Read the model definition and answer for the solid it produces. Units are mm, in the model's axes. A direction names the side the tool comes from. Coordinates: 2 decimals unless noted, no trailing zeros. Loops run counter-clockwise (first coordinate to the right, second up) from the corner with the lowest first, then second, coordinate; pieces in that order, holes last.
from build123d import *

# Parameters (mm, degrees)
CYLINDER004_R          = 1.5
CYLINDER004_DEPTH      = 10
CYLINDER004_ROLL_ANGLE = 90
CYLINDER003_R          = 1.5
CYLINDER003_DEPTH      = 10
CYLINDER003_ROLL_ANGLE = 90
BOX016_W               = 22.5
BOX016_H               = 13
BOX016_DEPTH           = 13
BOX015_W               = 38
BOX015_H               = 10
BOX015_DEPTH           = 13
BOX013_W               = 98.5
BOX013_H               = 62
BOX013_DEPTH           = 10
BOX012_W               = 114.5
BOX012_H               = 66
BOX012_DEPTH           = 4
BOX014_W               = 118.5
BOX014_H               = 70
BOX014_DEPTH           = 5
BOX010_W               = 2
BOX010_H               = 10
BOX010_DEPTH           = 8
BOX010_PLACEMENT_ANGLE = 59
BOX011_W               = 2
BOX011_H               = 10
BOX011_DEPTH           = 8
BOX011_PLACEMENT_ANGLE = 59
BOX009_W               = 2
BOX009_H               = 10
BOX009_DEPTH           = 8
BOX009_PLACEMENT_ANGLE = 59
BOX008_W               = 2
BOX008_H               = 10
BOX008_DEPTH           = 8
BOX008_PLACEMENT_ANGLE = 59
BOX007_W               = 10
BOX007_H               = 45
BOX007_DEPTH           = 50
BOX006_W               = 14
BOX006_H               = 12
BOX006_DEPTH           = 12
BOX006_PLACEMENT_ANGLE = 59
BOX004_W               = 14
BOX004_H               = 12
BOX004_DEPTH           = 12
BOX004_PLACEMENT_ANGLE = 59
BOX002_W               = 71
BOX002_H               = 10
BOX002_DEPTH           = 25
BOX001_W               = 80
BOX001_H               = 30
BOX001_DEPTH           = 50
BOX_W                  = 84
BOX_H                  = 30
BOX_DEPTH              = 70
CYLINDER001_R          = 70
CYLINDER001_DEPTH      = 87
CYLINDER_R             = 72.5
CYLINDER_DEPTH         = 80
CYLINDER002_R          = 68
CYLINDER002_DEPTH      = 85


with BuildPart() as screwcutout002:
    # Cylinder004 → Cylinder004 (new body)
    with BuildSketch(Plane.XY):
        Circle(CYLINDER004_R)
    extrude(amount=CYLINDER004_DEPTH)


with BuildPart() as screwcutout002_1:
    # Cylinder004 roll: moved
    add(screwcutout002.part.rotate(Axis((0, 0, 0), (1, 0, 0)), CYLINDER004_ROLL_ANGLE))


with BuildPart() as screwcutout002_2:
    # Cylinder004 placement: moved
    add(screwcutout002_1.part.moved(Location((-15, 73, 14.5))))


with BuildPart() as screwcutout1:
    # Cylinder003 → Cylinder003 (new body)
    with BuildSketch(Plane.XY):
        Circle(CYLINDER003_R)
    extrude(amount=CYLINDER003_DEPTH)


with BuildPart() as screwcutout1_1:
    # Cylinder003 roll: moved
    add(screwcutout1.part.rotate(Axis((0, 0, 0), (1, 0, 0)), CYLINDER003_ROLL_ANGLE))


with BuildPart() as screwcutout1_2:
    # Cylinder003 placement: moved
    add(screwcutout1_1.part.moved(Location((15, 73, 14.5))))


with BuildPart() as powercutout:
    # Box016 → Box016 (new body)
    with BuildSketch(Plane(origin=(-11.25, 63, 8), x_dir=(1, 0, 0), z_dir=(0, 0, 1))):
        with Locations((11.25, 6.5)):
            Rectangle(BOX016_W, BOX016_H)
    extrude(amount=BOX016_DEPTH)


with BuildPart() as powerswitch:
    # Box015 → Box015 (new body)
    with BuildSketch(Plane(origin=(-19, 70, 8), x_dir=(1, 0, 0), z_dir=(0, 0, 1))):
        with Locations((19, 5)):
            Rectangle(BOX015_W, BOX015_H)
    extrude(amount=BOX015_DEPTH)


with BuildPart() as battery_cutout:
    # Box013 → Box013 (new body)
    with BuildSketch(Plane(origin=(-44, -31, 0), x_dir=(1, 0, 0), z_dir=(0, 0, 1))):
        with Locations((49.25, 31)):
            Rectangle(BOX013_W, BOX013_H)
    extrude(amount=BOX013_DEPTH)


with BuildPart() as battery_cutout001:
    # Box012 → Box012 (new body)
    with BuildSketch(Plane(origin=(-58, -33, 0), x_dir=(1, 0, 0), z_dir=(0, 0, 1))):
        with Locations((57.25, 33)):
            Rectangle(BOX012_W, BOX012_H)
    extrude(amount=BOX012_DEPTH)


with BuildPart() as obj1:
    # Box014 → Box014 (new body)
    with BuildSketch(Plane(origin=(-60, -35, 0), x_dir=(1, 0, 0), z_dir=(0, 0, 1))):
        with Locations((59.25, 35)):
            Rectangle(BOX014_W, BOX014_H)
    extrude(amount=BOX014_DEPTH)


with BuildPart() as pin2_cutout001:
    # Box010 → Box010 (new body)
    with BuildSketch(Plane.XY):
        with Locations((1, 5)):
            Rectangle(BOX010_W, BOX010_H)
    extrude(amount=BOX010_DEPTH)


with BuildPart() as pin2_cutout001_1:
    # Box010 placement: moved
    add(pin2_cutout001.part.moved(Location((67, -33, 45))).rotate(Axis((67, -33, 45), (0, 0, 1)), BOX010_PLACEMENT_ANGLE))


with BuildPart() as pin1_cutout001:
    # Box011 → Box011 (new body)
    with BuildSketch(Plane.XY):
        with Locations((1, 5)):
            Rectangle(BOX011_W, BOX011_H)
    extrude(amount=BOX011_DEPTH)


with BuildPart() as pin1_cutout001_1:
    # Box011 placement: moved
    add(pin1_cutout001.part.moved(Location((62, -44, 45))).rotate(Axis((62, -44, 45), (0, 0, 1)), BOX011_PLACEMENT_ANGLE))


with BuildPart() as pin2_cutout:
    # Box009 → Box009 (new body)
    with BuildSketch(Plane.XY):
        with Locations((1, 5)):
            Rectangle(BOX009_W, BOX009_H)
    extrude(amount=BOX009_DEPTH)


with BuildPart() as pin2_cutout_1:
    # Box009 placement: moved
    add(pin2_cutout.part.moved(Location((67, -33, 27))).rotate(Axis((67, -33, 27), (0, 0, 1)), BOX009_PLACEMENT_ANGLE))


with BuildPart() as pin1_cutout:
    # Box008 → Box008 (new body)
    with BuildSketch(Plane.XY):
        with Locations((1, 5)):
            Rectangle(BOX008_W, BOX008_H)
    extrude(amount=BOX008_DEPTH)


with BuildPart() as pin1_cutout_1:
    # Box008 placement: moved
    add(pin1_cutout.part.moved(Location((62, -44, 27))).rotate(Axis((62, -44, 27), (0, 0, 1)), BOX008_PLACEMENT_ANGLE))


with BuildPart() as rfid_cutout:
    # Box007 → Box007 (new body)
    with BuildSketch(Plane(origin=(-79, -22.5, 15), x_dir=(1, 0, 0), z_dir=(0, 0, 1))):
        with Locations((5, 22.5)):
            Rectangle(BOX007_W, BOX007_H)
    extrude(amount=BOX007_DEPTH)


with BuildPart() as box006:
    # Box006 → Box006 (new body)
    with BuildSketch(Plane.XY):
        with Locations((7, 6)):
            Rectangle(BOX006_W, BOX006_H)
    extrude(amount=BOX006_DEPTH)


with BuildPart() as box006_1:
    # Box006 placement: moved
    add(box006.part.moved(Location((67, -47, 25))).rotate(Axis((67, -47, 25), (0, 0, 1)), BOX006_PLACEMENT_ANGLE))


with BuildPart() as box004:
    # Box004 → Box004 (new body)
    with BuildSketch(Plane.XY):
        with Locations((7, 6)):
            Rectangle(BOX004_W, BOX004_H)
    extrude(amount=BOX004_DEPTH)


with BuildPart() as box004_1:
    # Box004 placement: moved
    add(box004.part.moved(Location((67, -47, 43))).rotate(Axis((67, -47, 43), (0, 0, 1)), BOX004_PLACEMENT_ANGLE))


with BuildPart() as obj2:
    # Box002 → Box002 (new body)
    with BuildSketch(Plane(origin=(-35.5, -59, 27.5), x_dir=(1, 0, 0), z_dir=(0, 0, 1))):
        with Locations((35.5, 5)):
            Rectangle(BOX002_W, BOX002_H)
    extrude(amount=BOX002_DEPTH)


with BuildPart() as display_cutout_big:
    # Box001 → Box001 (new body)
    with BuildSketch(Plane(origin=(-40, -84.5, 15), x_dir=(1, 0, 0), z_dir=(0, 0, 1))):
        with Locations((40, 15)):
            Rectangle(BOX001_W, BOX001_H)
    extrude(amount=BOX001_DEPTH)


with BuildPart() as obj3:
    # Box → Box (new body)
    with BuildSketch(Plane(origin=(-42, -83.5, 0), x_dir=(1, 0, 0), z_dir=(0, 0, 1))):
        with Locations((42, 15)):
            Rectangle(BOX_W, BOX_H)
    extrude(amount=BOX_DEPTH)


with BuildPart() as wall:
    # Cylinder001 → Cylinder001 (new body)
    with BuildSketch(Plane.XY):
        Circle(CYLINDER001_R)
    extrude(amount=CYLINDER001_DEPTH)


with BuildPart() as fusion:
    # Cylinder → Cylinder (new body)
    with BuildSketch(Plane.XY):
        Circle(CYLINDER_R)
    extrude(amount=CYLINDER_DEPTH)

    # Fusion: union wall
    add(wall.part)


with BuildPart() as common:
    # Common base: copy of Fusion
    add(fusion.part)

    # Common: intersect obj3
    add(obj3.part, mode=Mode.INTERSECT)


with BuildPart() as base_cutout:
    # Cylinder002 → Cylinder002 (new body)
    with BuildSketch(Plane.XY.offset(2)):
        Circle(CYLINDER002_R)
    extrude(amount=CYLINDER002_DEPTH)


with BuildPart() as cut016:
    # Cut base: copy of Fusion
    add(fusion.part)

    # Cut: cut base_cutout
    add(base_cutout.part, mode=Mode.SUBTRACT)

    # Fusion001: union Common
    add(common.part)

    # Cut001: cut display_cutout_big
    add(display_cutout_big.part, mode=Mode.SUBTRACT)

    # Cut002: cut obj2
    add(obj2.part, mode=Mode.SUBTRACT)

    # Cut003: cut Box004
    add(box004_1.part, mode=Mode.SUBTRACT)

    # Cut004: cut Box006
    add(box006_1.part, mode=Mode.SUBTRACT)

    # Cut005: cut rfid_cutout
    add(rfid_cutout.part, mode=Mode.SUBTRACT)

    # Cut006: cut pin1_cutout
    add(pin1_cutout_1.part, mode=Mode.SUBTRACT)

    # Cut007: cut pin2_cutout
    add(pin2_cutout_1.part, mode=Mode.SUBTRACT)

    # Cut008: cut pin1_cutout001
    add(pin1_cutout001_1.part, mode=Mode.SUBTRACT)

    # Cut009: cut pin2_cutout001
    add(pin2_cutout001_1.part, mode=Mode.SUBTRACT)

    # Fusion002: union obj1
    add(obj1.part)

    # Cut010: cut battery_cutout001
    add(battery_cutout001.part, mode=Mode.SUBTRACT)

    # Cut011: cut battery_cutout
    add(battery_cutout.part, mode=Mode.SUBTRACT)

    # Cut012: cut PowerSwitch
    add(powerswitch.part, mode=Mode.SUBTRACT)

    # Cut013: cut PowerSwitch
    add(powerswitch.part, mode=Mode.SUBTRACT)

    # Cut014: cut PowerCutout
    add(powercutout.part, mode=Mode.SUBTRACT)

    # Cut015: cut ScrewCutout1
    add(screwcutout1_2.part, mode=Mode.SUBTRACT)

    # Cut016: cut ScrewCutout002
    add(screwcutout002_2.part, mode=Mode.SUBTRACT)


solid = cut016.part
Q1. A cutting plane is placed at C-C (y = 20). Give the vertices of the cut face in (x, z), then the cut area to 3 significant figures.
Findings below:
outline: (-69.69, 0) - (-58, 0) - (-58, 4) - (-44, 4) - (-44, 5) - (-60, 5) - (-60, 2) - (-64.99, 2) - (-64.99, 87) - (-67.08, 87) - (-67.08, 80) - (-69.69, 80) - (-69.69, 65) - (-69, 65) - (-69, 15) - (-69.69, 15) - close; (54.5, 4) - (56.5, 4) - (56.5, 0) - (69.69, 0) - (69.69, 80) - (67.08, 80) - (67.08, 87) - (64.99, 87) - (64.99, 2) - (58.5, 2) - (58.5, 5) - (54.5, 5) - close
area: 805 mm2
Q2. Straight lines are drawn through the part: probe 1 along Z at (x, y) = (-15, 68.05); probe 2 along Z at (x, y) = (-45, 10); probe 3 along Y at (x, z) = (50.5, 73). For each, find the intervals that lie inside material, in ascending order.
Findings below:
probe 1: z = 0 to 13, 16 to 87
probe 2: z = 4 to 5
probe 3: y = -52.02 to -45.54, 45.54 to 52.02
Q3. Which of the six approach directions +Z, -Z, +X, -X, +Y, -Y give full straight-line access (tool end or side, diameter ignored) to faces 4 (the face through (-48, 0, 4)), 5 (the face through (-23, 31.3, 5)), 6 (the face through (-40, -58, 40)), 7 (the face through (-14, 70, 13))?
Findings below:
face 4: -Z
face 5: +Z
face 6: -Y
face 7: +X, -X, +Y
Q4. A cutting plane is placed at D-D (y = 38). Give the vertices of the cut face in (x, z), then the cut area to 3 significant figures.
Findings below:
outline: (-61.74, 0) - (61.74, 0) - (61.74, 80) - (58.79, 80) - (58.79, 87) - (56.39, 87) - (56.39, 2) - (-56.39, 2) - (-56.39, 87) - (-58.79, 87) - (-58.79, 80) - (-61.74, 80) - close
area: 1,120 mm2
Q5. A cutting plane is placed at B-B (x = 0). Count the separate pieces of the cut face and the enclosed holes in it, then the cut area to 4 significant figures.
Findings below:
separate pieces: 4
enclosed holes: 0
area: 906.5 mm2
Q6. A cutting plane is placed at A-A (z = 62.5). Give the vertices of the cut face in (x, y), then the cut area to 3 significant figures.
Findings below:
outline: (-69, -22.25) arc R72.5 ccw to (-40, -60.47) - (-40, -54.5) - (40, -54.5) - (40, -60.47) arc R72.5 ccw (long way) to (-69, 22.25) - close; hole (-41.97, -53.5) - (41.97, -53.5) arc R68 ccw (long way) to start
area: 1,580 mm2
Q7. Determine the mould class of faces 1 (the face through (-38, 59, 80)), 2 (the face through (-1, -61, 15)), 3 (the face through (56.5, 0, 2)) for opening direction Z: +Z half, -Z half, draft (parallel to the pull), parting line (faces both ways), or undercut.
Findings below:
face 1: +Z half
face 2: undercut
face 3: draft
Q8. Flat-ended cylindrical pins translate along their axes: pin 1 Ø3 at (x, z) = (1, 2.5) entering from -Y; pin 2 Ø0.5 at (y, z) = (-54, 44) entering from -X; pin 3 Ø2.5 at (x, z) = (15, 14.5) entering from +Y; pin 4 Ø6 at (x, y) = (-38.5, -27) entering from +Z. Find the tip coordinate at first contact, or state that the pin passes through.
Findings below:
pin 1: stops at y = -72.5
pin 2: stops at x = -48.65
pin 3: stops at y = -53.5
pin 4: passes through
